For this review, take the finished solid that the model builds, in its own axes (mm). Face numbers are marked on the shaded views. Round coordinates to 2 decimals unless told otherwise and drop trailing zeros. Order: outer loops, then holes, each group sorted by start corner. A loop starts at its lowest first (then second) coordinate and runs counter-clockwise, first axis right, second up. Notation, with made-up numbers: (-0.75, 63.5) - (14.25, 63.5) arc R28 ccw to (14.25, 85.5) - close; hole circle Ø5 at (37, -12.5). An arc over 180 degrees is marked (long way). One line per question, with ' | ' between items.
```python
from build123d import *

# Parameters (mm, degrees)
F_1_4_0_25_DIAMETER_HOLE1_REACH  = 380.534
F_1_4_0_25_DIAMETER_HOLE1_BORE_R = 3.175
CIRPATTERN2_COUNT                = 4
CHAMFER1_SIZE                    = 1.27
CIRPATTERN1_COUNT                = 6
SKETCH7_W                        = 14.732
SKETCH7_H                        = 14.732
CUT_EXTRUDE1_DEPTH               = 0.635
SKETCH8_W                        = 16.51
SKETCH8_H                        = 16.51
CUT_EXTRUDE2_DEPTH               = 0.635
CIRPATTERN4_COUNT                = 6
CIRPATTERN5_COUNT                = 4


with BuildPart() as part:
    # Sketch2 → Revolve1 (revolve)
    with BuildSketch(Plane.XY, mode=Mode.PRIVATE) as revolve1_sk:
        Polygon((41.275, 0), (44.45, 0), (44.45, 372.618), (41.275, 372.618), (41.275, 186.309), align=None)
    revolve(revolve1_sk.sketch.rotate(Axis((0, 0, 0), (0, 1, 0)), 90), axis=Axis((0, 0, 0), (0, 1, 0)))

    # 1/4 (0.25) Diameter Hole1 bore (on position points) → 1/4 (0.25) Diameter Hole1 (cut, up to next)
    with BuildSketch(Plane(origin=(0, 7.366, -44.45), x_dir=(-1, 0, 0), z_dir=(0, 0, -1)), mode=Mode.PRIVATE) as f_1_4_0_25_diameter_hole1_sk1:
        Circle(F_1_4_0_25_DIAMETER_HOLE1_BORE_R)
    f_1_4_0_25_diameter_hole1_tool1 = extrude(f_1_4_0_25_diameter_hole1_sk1.sketch, amount=-F_1_4_0_25_DIAMETER_HOLE1_REACH, mode=Mode.PRIVATE) & part.part
    f_1_4_0_25_diameter_hole1 = f_1_4_0_25_diameter_hole1_tool1.solids().sort_by_distance((0, 7.366, -44.45))[0]
    add(f_1_4_0_25_diameter_hole1, mode=Mode.SUBTRACT)

    # Sketch6 → 1/4 (0.25) Diameter Hole2 (revolve, cut)
    with BuildSketch(Plane(origin=(0, 366.268, -44.45), x_dir=(0, 1, 0), z_dir=(1, 0, 0))):
        Polygon((0, 0), (0, 5.209732465), (3.175, 3.302), (3.175, 0), align=None)
    f_1_4_0_25_diameter_hole2 = revolve(axis=Axis((0, 366.268, -50.8), (0, 0, 1)), mode=Mode.SUBTRACT)

    # CirPattern2: 1/4 (0.25) Diameter Hole2 ×4 about axis
    cirpattern2_axis = Axis((0, -17.04721, 0), (0, 1, 0))
    for i in range(1, CIRPATTERN2_COUNT):
        add(f_1_4_0_25_diameter_hole2.rotate(cirpattern2_axis, i * 360 / CIRPATTERN2_COUNT), mode=Mode.SUBTRACT)

    # Chamfer1
    chamfer1_edges = [part.edges().sort_by_distance(p)[0] for p in [
        (0, 372.618, 41.275),
        (0, 0, 41.275),
    ]]
    chamfer(chamfer1_edges, length=CHAMFER1_SIZE)

    # CirPattern1: 1/4 (0.25) Diameter Hole1 ×6 about axis
    cirpattern1_axis = Axis((0, -17.04721, 0), (0, 1, 0))
    for i in range(1, CIRPATTERN1_COUNT):
        add(f_1_4_0_25_diameter_hole1.rotate(cirpattern1_axis, i * 360 / CIRPATTERN1_COUNT), mode=Mode.SUBTRACT)

    # Sketch7 → Cut-Extrude1 (cut)
    with BuildSketch(Plane(origin=(0, 0, -44.45), x_dir=(-1, 0, 0), z_dir=(0, 0, -1))):
        with Locations((0, 7.366)):
            Rectangle(SKETCH7_W, SKETCH7_H)
    cut_extrude1 = extrude(amount=-CUT_EXTRUDE1_DEPTH, mode=Mode.SUBTRACT)

    # Sketch8 → Cut-Extrude2 (cut)
    with BuildSketch(Plane(origin=(0, 0, -44.45), x_dir=(-1, 0, 0), z_dir=(0, 0, -1))):
        with Locations((0, 366.268)):
            Rectangle(SKETCH8_W, SKETCH8_H)
    cut_extrude2 = extrude(amount=-CUT_EXTRUDE2_DEPTH, mode=Mode.SUBTRACT)

    # CirPattern4: Cut-Extrude1 ×6 about axis
    cirpattern4_axis = Axis((0, 0, 0), (0, 1, 0))
    for i in range(1, CIRPATTERN4_COUNT):
        add(cut_extrude1.rotate(cirpattern4_axis, i * 360 / CIRPATTERN4_COUNT), mode=Mode.SUBTRACT)

    # CirPattern5: Cut-Extrude2 ×4 about axis
    cirpattern5_axis = Axis((0, 0, 0), (0, 1, 0))
    for i in range(1, CIRPATTERN5_COUNT):
        add(cut_extrude2.rotate(cirpattern5_axis, i * 360 / CIRPATTERN5_COUNT), mode=Mode.SUBTRACT)


solid = part.part
```
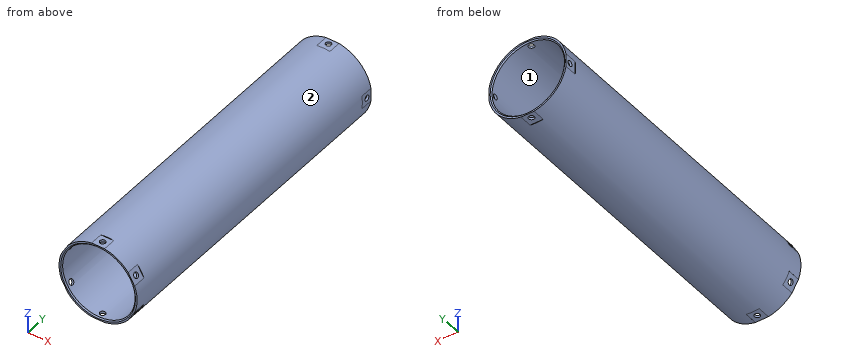
(1) Insertion check: pin 1 (6 mm diameter, centred on y = 211.5, z = -28.5, fed in from -X); pin 2 (10 mm diameter, centred on y = 366.268, z = 0, fed in from -X) (3 decimals); pin 3 (2 mm diameter, centred on x = -32, y = 288.5, fed in from +Z). Each pin has a flat end and moves straight along its axis. Give the tip position at first contact, or say it passes through.
Output values:
pin 1: x = -36.41 | pin 2: x = -43.815 | pin 3: z = 31.86
(2) Mouldability with a two-part tool opening along Z and no side actions: class the marked faces 1 and 2 as released by +Z, released by -Z, zero draft, split by the parting line, or undercut.
Output values:
face 1: undercut | face 2: split by the parting line
(3) We need section B-B on x = 0. Give the number of separate pieces and of enclosed holes in the cut face, plus the area to 3 significant figures.
Output values:
separate pieces: 6 | enclosed holes: 0 | area: 2,260 mm^2
(4) We need section A-A on z = 0. State the section outline as (x, y) points (3 decimals), plus the area to 3 significant figures.
Output values:
outline: (-44.45, 0) - (-42.545, 0) - (-41.275, 1.27) - (-41.275, 363.093) - (-43.815, 363.093) - (-43.815, 358.013) - (-44.45, 358.013) - close; (-43.815, 369.443) - (-41.275, 369.443) - (-41.275, 371.348) - (-42.545, 372.618) - (-43.815, 372.618) - close; (41.275, 1.27) - (42.545, 0) - (44.45, 0) - (44.45, 358.013) - (43.815, 358.013) - (43.815, 363.093) - (41.275, 363.093) - close; (41.275, 369.443) - (43.815, 369.443) - (43.815, 372.618) - (42.545, 372.618) - (41.275, 371.348) - close | area: 2,310 mm^2
(5) We need section C-C on y = 206. State the section outline as (x, z) points (3 decimals).
Output values:
outline: circle Ø88.9 at (0, 0); hole circle Ø82.55 at (0, 0)
(6) For probe 1 along Y at (x, z) = (0, 41.7) (3 decimals); probe 2 along Y at (x, z) = (0, 42.1) (3 decimals); probe 3 along X at (y, z) = (91, 6), list the stretches that pass through material, from the lowest coordinate up. Write a range as [from, to].
Output values:
probe 1: [0.845, 4.191], [10.541, 363.093], [369.443, 371.773] | probe 2: [0.445, 4.191], [10.541, 363.093], [369.443, 372.173] | probe 3: [-44.04, -40.84], [40.84, 44.04]
